For this review, take the finished solid that the model builds, in its own axes (mm). Face numbers are marked on the shaded views. A direction names the side the tool comes from. Coordinates: 2 decimals unless noted, no trailing zeros. Write each loop counter-clockwise with the first axis right and the second up, starting at its lowest first coordinate (ties: lowest second). Pieces come first, ordered by that corner, then holes. Notation, with made-up numbers: M 76,73.5 L 87,73.5 A16 cw 87,89.5 Z; hole C 20.5,23 d4. An arc over 180 degrees is marked long. Return JSON: item names as keys, results as strings.
```python
from build123d import *

# Parameters (mm, degrees)
SKETCH1_W           = 43
SKETCH1_H           = 30
BOSS_EXTRUDE1_DEPTH = 36
SKETCH2_W           = 30
SKETCH2_H           = 11
CUT_EXTRUDE1_DEPTH  = 30
SKETCH3_R           = 11.15
CUT_EXTRUDE2_DEPTH  = 7
CUT_EXTRUDE3_START  = -7
SKETCH4_R           = 11.15
CUT_EXTRUDE3_DEPTH  = 7
SKETCH5_R           = 9.5
CUT_EXTRUDE4_DEPTH  = 40.092838219
FILLET2_R           = 15
SKETCH6_W           = 30
SKETCH6_H           = 70
BOSS_EXTRUDE2_DEPTH = 10
SKETCH7_W           = 30
SKETCH7_H           = 15
BOSS_EXTRUDE3_DEPTH = 7
SKETCH8_R           = 4.15
CUT_EXTRUDE5_DEPTH  = 70.878465925
SKETCH9_R           = 8
CUT_EXTRUDE6_DEPTH  = 77.439518575
BOSS_EXTRUDE4_START = 5
SKETCH10_W          = 30
SKETCH10_H          = 17
SKETCH10_R          = 4.15
BOSS_EXTRUDE4_DEPTH = 5


with BuildPart() as part:
    # Sketch1 → Boss-Extrude1 (new body)
    with BuildSketch(Plane(origin=(0, 0, 0), x_dir=(1, 0, 0), z_dir=(0, 1, 0))):
        Rectangle(SKETCH1_W, SKETCH1_H)
    extrude(amount=BOSS_EXTRUDE1_DEPTH)

    # Sketch2 → Cut-Extrude1 (cut)
    with BuildSketch(Plane.ZY.offset(21.5)):
        with Locations((0, 18)):
            Rectangle(SKETCH2_W, SKETCH2_H)
    extrude(amount=-CUT_EXTRUDE1_DEPTH, mode=Mode.SUBTRACT)

    # Sketch3 → Cut-Extrude2 (cut)
    with BuildSketch(Plane(origin=(0, 36, 0), x_dir=(1, 0, 0), z_dir=(0, 1, 0))):
        with Locations(Location((-3.5, 0, 0), (0, 0, 270))):
            Circle(SKETCH3_R)
    extrude(amount=-CUT_EXTRUDE2_DEPTH, mode=Mode.SUBTRACT)

    # Sketch4 → Cut-Extrude3 (cut)
    with BuildSketch(Plane.XZ.offset(CUT_EXTRUDE3_START)):
        with Locations(Location((-3.5, 0, 0), (0, 0, 90))):
            Circle(SKETCH4_R)
    extrude(amount=CUT_EXTRUDE3_DEPTH, mode=Mode.SUBTRACT)

    # Sketch5 → Cut-Extrude4 (cut, through all)
    with BuildSketch(Plane(origin=(0, 29, 0), x_dir=(1, 0, 0), z_dir=(0, 1, 0))):
        with Locations(Location((-3.5, 0, 0), (0, 0, 90))):
            Circle(SKETCH5_R)
    extrude(amount=-CUT_EXTRUDE4_DEPTH, mode=Mode.SUBTRACT)

    # Fillet2
    fillet2_edges = [part.edges().sort_by_distance(p)[0] for p in [
        (-21.5, 6.25, -15),
        (-21.5, 6.25, 15),
        (-21.5, 29.75, 15),
        (-21.5, 29.75, -15),
    ]]
    fillet(fillet2_edges, radius=FILLET2_R - 0.0001)  # a hair under: the kernel refuses the full size

    # Sketch6 → Boss-Extrude2 (add)
    with BuildSketch(Plane(origin=(21.5, 0, 0), x_dir=(0, 0, -1), z_dir=(1, 0, 0))):
        with Locations((0, 18)):
            Rectangle(SKETCH6_W, SKETCH6_H)
    extrude(amount=BOSS_EXTRUDE2_DEPTH)

    # Sketch7 → Boss-Extrude3 (add)
    with BuildSketch(Plane(origin=(31.5, 0, 0), x_dir=(0, 0, -1), z_dir=(1, 0, 0))):
        with Locations((0, 30.65)):
            Rectangle(SKETCH7_W, SKETCH7_H)
        with Locations((0, 5.25)):
            Rectangle(SKETCH7_W, SKETCH7_H)
    extrude(amount=BOSS_EXTRUDE3_DEPTH)

    # Sketch8 → Cut-Extrude5 (cut, through all)
    with BuildSketch(Plane.ZY.offset(-21.5)):
        with Locations((0, -8.5)):
            Circle(SKETCH8_R)
        with Locations((0, 44.5)):
            Circle(SKETCH8_R)
    extrude(amount=-CUT_EXTRUDE5_DEPTH, mode=Mode.SUBTRACT)

    # Sketch9 → Cut-Extrude6 (cut, through all)
    with BuildSketch(Plane(origin=(31.5, 0, 0), x_dir=(0, 0, -1), z_dir=(1, 0, 0))):
        with Locations((0, -8.5)):
            Circle(SKETCH9_R)
        with Locations((0, 44.5)):
            Circle(SKETCH9_R)
    extrude(amount=CUT_EXTRUDE6_DEPTH, mode=Mode.SUBTRACT)

    # Sketch10 → Boss-Extrude4 (add)
    # profile 1 of 2: a face of its own
    with BuildSketch(Plane.ZY.offset(-21.5).offset(BOSS_EXTRUDE4_START)):
        with Locations((0, -8.5)):
            Rectangle(SKETCH10_W, SKETCH10_H)
        with Locations((0, -8.5)):
            Circle(SKETCH10_R, mode=Mode.SUBTRACT)
    # profile 2 of 2: a face of its own
    with BuildSketch(Plane.ZY.offset(-21.5).offset(BOSS_EXTRUDE4_START)):
        with Locations((0, 44.5)):
            Rectangle(SKETCH10_W, SKETCH10_H)
        with Locations((0, 44.5)):
            Circle(SKETCH10_R, mode=Mode.SUBTRACT)
    extrude(amount=-BOSS_EXTRUDE4_DEPTH)


solid = part.part
```
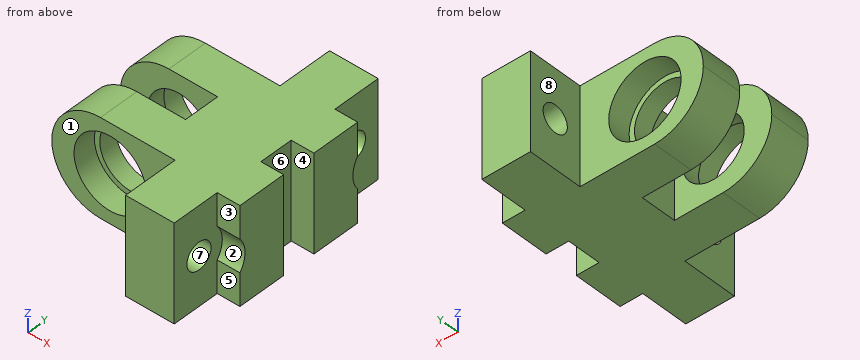
1. We need section C-C (x = 33.5). State the section outline as (y, z) points, plus the area to 3 significant figures.
Checks:
{"outline": "M -2.25,-15 L 12.75,-15 L 12.75,15 L -2.25,15 L -2.25,4.99 A8 cw -2.25,-4.99 Z; M 23.15,-15 L 38.15,-15 L 38.15,-4.87 A8 cw 38.15,4.87 L 38.15,15 L 23.15,15 Z", "area": "877 mm2"}
2. We need section D-D (y = -11). State the section outline as (x, z) points, plus the area to 3 significant figures.
Checks:
{"outline": "M 16.5,-15 L 31.5,-15 L 31.5,-3.31 L 16.5,-3.31 Z; M 16.5,3.31 L 31.5,3.31 L 31.5,15 L 16.5,15 Z", "area": "351 mm2"}
3. Draft analysis for pull direction Y (two halves, no side actions). For the marked faces 5, 6, 7 and 8, state which applies: +Y half, -Y half, draft (parallel to the pull), parting line (faces both ways), or undercut.
Checks:
{"face 5": "-Y half", "face 6": "undercut", "face 7": "undercut", "face 8": "draft"}
4. Clearance check with flat-ended pins moving along their axes: pin 1 Ø3.5 at (x, z) = (34.5, 8.5) entering from -Y; pin 2 Ø5 at (y, z) = (-6.5, -3) entering from +X; pin 3 Ø8.5 at (y, z) = (-4.5, 6.5) entering from -X. State where each tip first meets the part, or that it passes through.
Checks:
{"pin 1": "y = -2.25", "pin 2": "x = 31.5", "pin 3": "x = 16.5"}
5. We need section B-B (x = -3.5). State the section outline as (y, z) points, plus the area to 3 significant figures.
Checks:
{"outline": "M 0,-15 L 12.5,-15 L 12.5,-9.5 L 7,-9.5 L 7,-11.15 L 0,-11.15 Z; M 0,11.15 L 7,11.15 L 7,9.5 L 12.5,9.5 L 12.5,15 L 0,15 Z; M 23.5,-15 L 36,-15 L 36,-11.15 L 29,-11.15 L 29,-9.5 L 23.5,-9.5 Z; M 23.5,9.5 L 29,9.5 L 29,11.15 L 36,11.15 L 36,15 L 23.5,15 Z", "area": "229 mm2"}
6. For the marked faces 1, 2, 3 and 4, list the 3-axis set-ups (+Z, -Z, +X, -X, +Y, -Y) from which the entire face can be reached by the end or side of a thin tool; tool diameter is ignored.
Checks:
{"face 1": "+Z, -Z, -X, -Y", "face 2": "+X, -Y", "face 3": "+Z, -Z, +X, -Y", "face 4": "+Z, -Z, +X"}
7. Wall thickness on L1, parallel to Y at x = 35, z = 10.5; L2, parallel to X at y = 2, z = 0; L3, parallel to Y at x = -17, z = 4: over which ranges is each line inside the solid? List them lowest first. Write a range as from..to.
Checks:
{"L1": "-2.25..12.75, 23.15..38.15", "L2": "-21.5..-14.65, 7.65..38.5", "L3": "0..12.5, 23.5..36"}
